from build123d import *

# Parameters (mm, degrees)
F2_SIZE2 = 2
F2_SIZE  = 2
F3_R     = 4.652027
F4_DEPTH = 270.001
F6_R     = 6.482878
F7_DEPTH = 270.001


with BuildPart() as f1:
    # F0 (on Front) → F1 (revolve)
    with BuildSketch(Plane.XZ):
        with BuildLine():
            Line((-135, 30), (-135, 0))
            Line((-135, 0), (135, 0))
            Line((135, 0), (135, 15))
            Line((135, 15), (-63, 15))
            ThreePointArc((-63, 15), (-64.414214, 15.585786), (-65, 17))
            Line((-65, 17), (-65, 30))
            Line((-65, 30), (-135, 30))
        make_face()
    revolve(axis=Axis((9.817764, 0, 0), (1, 0, 0)))

    # F2
    f2_edges = [f1.edges().sort_by_distance(p)[0] for p in [
        (-65, 0, -30),
        (-135, 0, -30),
        (-100, 0, 30),
        (135, 0, -15),
    ]]
    chamfer(f2_edges, length=F2_SIZE, length2=F2_SIZE2)

    # F3 (on face) → F4 (cut, through all)
    with BuildSketch(Plane.YZ.offset(135)):
        Circle(F3_R)
    extrude(amount=-F4_DEPTH, mode=Mode.SUBTRACT)

    # F6 (on face) → F7 (cut, through all)
    with BuildSketch(Plane(origin=(-135, 0, 0), x_dir=(0, -1, 0), z_dir=(-1, 0, 0))):
        with Locations((7.74362, 10.037243)):
            Circle(F6_R)
    extrude(amount=-F7_DEPTH, mode=Mode.SUBTRACT)


solid = f1.part
Can you work these out from the model? Positions are in its coordinate system, mm. A direction names the side the tool comes from. Give positions to 0.01 mm unless a question says otherwise; leave off trailing zeros. Write each loop counter-clockwise with the first axis right and the second up, starting at its lowest first coordinate (ties: lowest second). Pieces come first, ordered by that corner, then holes. Notation, with made-up numbers: (15, 71) -> (33, 71) arc R23 cw to (33, 98) -> close; hole circle Ø11 at (50.25, 36). An arc over 180 degrees is marked (long way). Answer as a JSON object with one key per item and string values. Group by question number.
Item 1: Suppose I cut it at B-B (x = 37.5). Please give me the cut outline in (y, z), plus the area to 3 significant figures.
Item 2: Please list where these lines run through material, in increasing order: line 1 (Z direction, x = 19, y = 0); line 2 (X direction, y = -4.5, z = 16); line 3 (Y direction, x = 28.5, z = -1). Write a range as [from, to].
Item 3: For faces 1 (the face through (-134.87, 27.46, -6.1)), 2 (the face through (-65, 18, 0)), which set-ups out of +Z, -Z, +X, -X, +Y, -Y let a thin tool reach every point of the face, with its end or its side?
Item 4: We'd pull the mould along Y, two halves only. Please class faces 3 (the face through (135, 0, -6)), 4 (the face through (1.89, 4.437, 1.397)), 5 (the face through (-100.46, -1.32, -29.97)): +Y half, -Y half, draft (parallel to the pull), parting line (faces both ways), or undercut.
Item 5: I'm going to push flat-ended pins straight in: P1, Ø4, axis at x = -42, y = -4.5, coming from the -Z side; P2, Ø8, axis at x = 97, z = -17, coming from the +Y side; P3, Ø10, axis at x = 31.5, y = 16, coming from the +Z side. Where does each tip first touch, or does it pass through?
Item 6: Suppose I cut it at A-A (z = 0). Please give me the cut outline in (x, y), plus the area to 3 significant figures.
Findings:
{
 "1": {"outline": "(-13.37, 6.81) arc R15 ccw (long way) to (-3.19, 14.66) arc R6.48 cw (long way) to start; hole circle Ø9.3 at (0, 0)", "area": "549 mm²"},
 "2": {"line 1": "z = [-15, -4.65], [4.65, 15]", "line 2": "x = [-135, -64.96]", "line 3": "y = [-14.97, -4.54], [4.54, 14.97]"},
 "3": {"face 1": "-X", "face 2": "+X"},
 "4": {"face 3": "draft", "face 4": "undercut", "face 5": "parting line"},
 "5": {"P1": "stops at z = -14.79", "P2": "stops at y = 7.48", "P3": "stops at z = 10.2"},
 "6": {"outline": "(-135, -28) -> (-133, -30) -> (-67, -30) -> (-65, -28) -> (-65, -17) arc R2 cw to (-63, -15) -> (133, -15) -> (135, -13) -> (135, -4.65) -> (-135, -4.65) -> close; (-135, 4.65) -> (135, 4.65) -> (135, 13) -> (133, 15) -> (-63, 15) arc R2 cw to (-65, 17) -> (-65, 28) -> (-67, 30) -> (-133, 30) -> (-135, 28) -> close", "area": "7,680 mm²"}
}
